Check sheet for the modelled part. Datum: model origin and axes. Units: mm. A direction names the side the tool comes from. Round coordinates to 2 decimals unless told otherwise and drop trailing zeros. Order: outer loops, then holes, each group sorted by start corner. A loop starts at its lowest first (then second) coordinate and runs counter-clockwise, first axis right, second up.
Q1. Mould release check, pull along X, two halves, no side actions. Record for faces 1 (the cylindrical face through (11.017, 1.252, -5.543)), 2 (the flat face through (0, 1, 12.065)), 3 (the cylindrical face through (11.017, 1.252, 5.391)), 4 (the flat face through (-16.51, 1, 0)): +X half, -X half, draft (parallel to the pull), parting line (faces both ways), or undercut.
Q2. Cross-section at A-A on z = 0. Record the cut outline in (x, y) (3 decimals).
Q3. Cross-section at D-D on y = 7. Record the cut outline in (x, z) (3 decimals).
Q4. Set-up check for faces 5 (the cylindrical face through (1.93, 5.67, 2.52)), 6 (the flat face through (0, 8.89, 0)): record each of +Z, -Z, +X, -X, +Y, -Y from which the full face is reachable in a straight line by a thin tool's end or side.
Q5. Scan lines: probe 1 along Y at (x, z) = (11, 2.25); probe 2 along X at (y, z) = (5.25, -1.5); probe 3 along X at (y, z) = (1.5, 4.5). Record each from-to range of solid material in increasing order.
Q6. Depth check by flat-ended pin: P1, Ø1, axis at x = -0.5, y = 7.5, coming from the +Z side (3 decimals); P2, Ø12, axis at x = 5, z = -9.5, coming from the +Y side; P3, Ø1, axis at y = 7, z = -2.5, coming from the -X side. Enter the tip coordinate at first touch or a pass-through.
Q7. Cross-section at B-B on x = 0. Record the cut outline in (y, z) (3 decimals), then the cut area to 3 significant figures.
Q8. Cross-section at C-C on z = -4.75. Record the cut outline in (x, y).
from build123d import *

# Parameters (mm, degrees)
SKETCH1_W             = 33.02
SKETCH1_H             = 24.13
BOSS_EXTRUDE1_DEPTH   = 2.54
SKETCH2_R             = 3.175
BOSS_EXTRUDE2_DEPTH   = 6.35
F_4_CLEARANCE_HOLE1_D = 3.4544


with BuildPart() as part:
    # Sketch1 → Boss-Extrude1 (new body)
    with BuildSketch(Plane(origin=(0, 0, 0), x_dir=(1, 0, 0), z_dir=(0, 1, 0))):
        Rectangle(SKETCH1_W, SKETCH1_H)
    extrude(amount=BOSS_EXTRUDE1_DEPTH)

    # Sketch2 → Boss-Extrude2 (add)
    with BuildSketch(Plane(origin=(0, 2.54, 0), x_dir=(1, 0, 0), z_dir=(0, 1, 0))):
        with Locations(Location((0, 0, 0), (0, 0, 90))):
            Circle(SKETCH2_R)
    extrude(amount=BOSS_EXTRUDE2_DEPTH)

    # #4 Clearance Hole1 (through all)
    with Locations(Plane(origin=(0, 2.54, 0), x_dir=(1, 0, 0), z_dir=(0, 1, 0))):
        with Locations((9.291486619, 5.466660474), (9.291486619, -5.466660474)):
            Hole(F_4_CLEARANCE_HOLE1_D / 2)


solid = part.part
Results found:
1. face 1: undercut
1. face 2: draft
1. face 3: undercut
1. face 4: -X half
2. outline: (-16.51, 0) - (16.51, 0) - (16.51, 2.54) - (3.175, 2.54) - (3.175, 8.89) - (-3.175, 8.89) - (-3.175, 2.54) - (-16.51, 2.54) - close
3. outline: circle Ø6.35 at (0, 0)
4. face 5: +Y
4. face 6: +Z, -Z, +X, -X, +Y
5. probe 1: y = 0 to 2.54
5. probe 2: x = -2.8 to 2.8
5. probe 3: x = -16.51 to 7.86, 10.72 to 16.51
6. P1: stops at z = 3.175
6. P2: stops at y = 2.54
6. P3: stops at x = -2.47
7. outline: (0, -12.065) - (2.54, -12.065) - (2.54, -3.175) - (8.89, -3.175) - (8.89, 3.175) - (2.54, 3.175) - (2.54, 12.065) - (0, 12.065) - close
7. area: 102 mm2
8. outline: (-16.51, 0) - (7.72, 0) - (7.72, 2.54) - (-16.51, 2.54) - close; (10.86, 0) - (16.51, 0) - (16.51, 2.54) - (10.86, 2.54) - close
